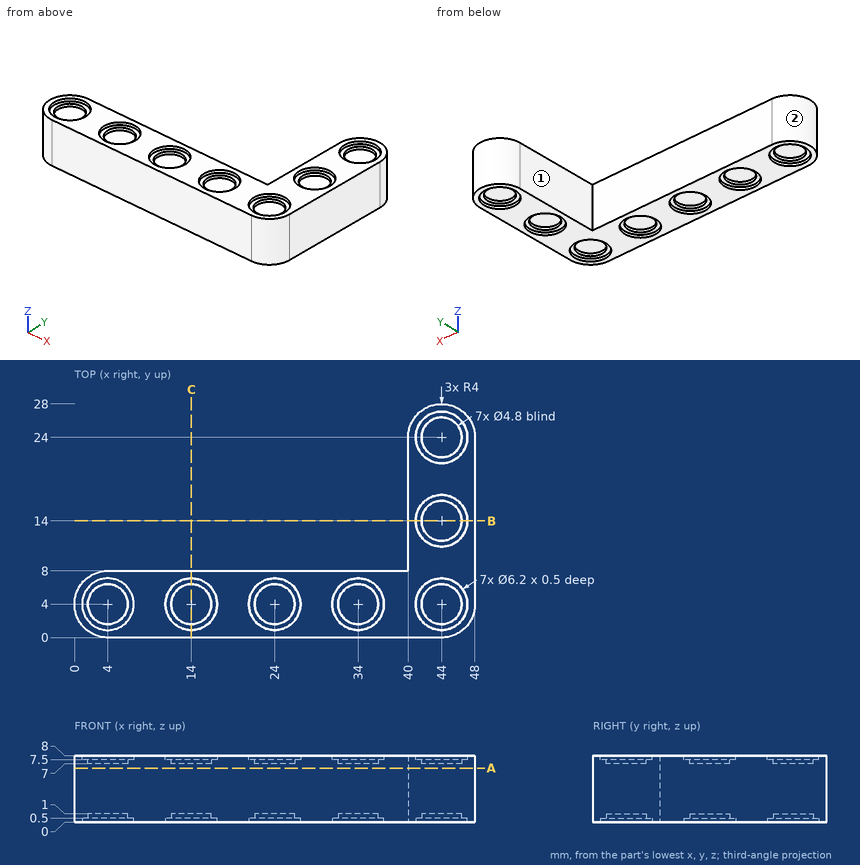
The drawing under review shows one solid part. Ordinate dimensions are in mm from its lowest x, y, z. A direction names the side the tool comes from. Coordinates: 2 decimals unless noted, no trailing zeros. Loops run counter-clockwise (first coordinate to the right, second up) from the corner with the lowest first, then second, coordinate; pieces in that order, holes last. Notation, with made-up numbers: (4, 82.25) -> (18, 82.25) arc R6 ccw to (18, 88.25) -> close; hole circle Ø6 at (81, 29.5). An arc over 180 degrees is marked (long way). Answer as a JSON object with one key per item and string values.
Q1. Clearance check with flat-ended pins moving along their axes: pin 1 Ø4 at (x, y) = (23, 3) entering from -Z; pin 2 Ø4 at (x, y) = (4, 4) entering from -Z; pin 3 Ø5 at (x, y) = (44, 4) entering from +Z; pin 4 Ø3 at (x, y) = (44, 14) entering from +Z. State where each tip first meets the part, or that it passes through.
Answer block:
{"pin 1": "stops at z = 0", "pin 2": "stops at z = 1", "pin 3": "stops at z = 7.5", "pin 4": "stops at z = 7"}
Q2. Take a section at B-B on y = 14. Give the boundary of the cut face in (x, z).
Answer block:
{"outline": "(40, 0) -> (40.9, 0) -> (40.9, 0.5) -> (41.6, 0.5) -> (41.6, 1) -> (46.4, 1) -> (46.4, 0.5) -> (47.1, 0.5) -> (47.1, 0) -> (48, 0) -> (48, 8) -> (47.1, 8) -> (47.1, 7.5) -> (46.4, 7.5) -> (46.4, 7) -> (41.6, 7) -> (41.6, 7.5) -> (40.9, 7.5) -> (40.9, 8) -> (40, 8) -> close"}
Q3. Tool access review of the marked faces 1 and 2: name each direction out of +Z, -Z, +X, -X, +Y, -Y from which nothing blocks a thin tool from reaching the whole face with its end or side.
Answer block:
{"face 1": "+Z, -Z, -X, +Y", "face 2": "+Z, -Z, -X"}
Q4. Take a section at A-A on z = 6.5. Give the boundary of the cut face in (x, y), plus the area to 3 significant figures.
Answer block:
{"outline": "(4, 0) -> (44, 0) arc R4 ccw to (48, 4) -> (48, 24) arc R4 ccw to (40, 24) -> (40, 8) -> (4, 8) arc R4 ccw to start", "area": "527 mm^2"}
Q5. To check wall thickness, follow L1, parallel to Y at x = 44, z = 0.2; L2, parallel to Y at x = 44, z = 7.25; L3, parallel to Y at x = 4, z = 7.2. State the ranges of each line that lie inside material, in increasing order.
Answer block:
{"L1": "y = 0 to 0.9, 7.1 to 10.9, 17.1 to 20.9, 27.1 to 28", "L2": "y = 0 to 1.6, 6.4 to 11.6, 16.4 to 21.6, 26.4 to 28", "L3": "y = 0 to 1.6, 6.4 to 8"}
Q6. Take a section at C-C on x = 14. Give the boundary of the cut face in (y, z).
Answer block:
{"outline": "(0, 0) -> (0.9, 0) -> (0.9, 0.5) -> (1.6, 0.5) -> (1.6, 1) -> (6.4, 1) -> (6.4, 0.5) -> (7.1, 0.5) -> (7.1, 0) -> (8, 0) -> (8, 8) -> (7.1, 8) -> (7.1, 7.5) -> (6.4, 7.5) -> (6.4, 7) -> (1.6, 7) -> (1.6, 7.5) -> (0.9, 7.5) -> (0.9, 8) -> (0, 8) -> close"}
